```python
from build123d import *

# Parameters (mm, degrees)
F1_DEPTH  = 40
F3_DEPTH  = 30
F4_DEPTH  = 13.8188209357
F6_DEPTH  = 20
F7_R      = 14
F8_DEPTH  = 20
F9_R      = 14
F10_DEPTH = 20


with BuildPart() as f1:
    # F0 (on Top) → F1 (new body)
    with BuildSketch(Plane.XY):
        Polygon((17.6335575688, -24.2705098312), (0, 0), (-30, 0), (-30, -15), (-7.6428817424, -15), (5.4983026531, -33.0872886156), align=None)
        Polygon((9.2705098312, 28.5316954889), (0, 0), (17.6335575688, -24.2705098312), (29.7688124844, -15.4537310469), (16.6276280888, 2.6335575688), (23.5363575757, 23.8964405732), align=None)
        Polygon((-30, 0), (0, 0), (9.2705098312, 28.5316954889), (-4.9953379132, 33.1669504045), (-10.8981379201, 15), (-30, 15), align=None)
    extrude(amount=F1_DEPTH)

    # F2 (on face) → F3 (cut, through all)
    with BuildSketch(Plane(origin=(12.1352549156, 8.8167787844, 0), x_dir=(-0.5877852523, 0.8090169944, 0), z_dir=(0.8090169944, 0.5877852523, 0))):
        Polygon((-30, 26.1811790643), (-7.6428817424, 40), (-30, 40), align=None)
        Polygon((-18.2909047095, 7.2373321675), (-30, 26.1811790643), (-30, 0), (-7.6428817424, 0), (-7.6428817424, 13.8188209357), align=None)
    extrude(amount=-F3_DEPTH, mode=Mode.SUBTRACT)

    # F4 (cut, through all): a face of the model
    f4_faces = [f1.faces().sort_by_distance(p)[0] for p in [
        (-5.1613250879, 7.1039545366, 0),
    ]]
    extrude(f4_faces, amount=-F4_DEPTH, mode=Mode.SUBTRACT)

    # F5 (on face) → F6 (cut)
    with BuildSketch(Plane(origin=(5.8766333563, -8.0884919048, -6.1796670384), x_dir=(0.8660332683, 0.3973019791, 0.303541621), z_dir=(0.4999863781, -0.6881722113, -0.5257686082))):
        with BuildLine():
            ThreePointArc((13.555551142, 11.7065510585), (20.8125243081, 16.7507031763), (23.6020646696, 25.1367388722))
            ThreePointArc((23.6020646696, 25.1367388722), (23.0669801184, 28.9702818755), (21.5026286756, 32.5107863592))
            Line((21.5026286756, 32.5107863592), (5.6485781973, 38.566926686))
            ThreePointArc((5.6485781973, 38.566926686), (-3.4762295905, 30.1325590497), (-2.2984993363, 17.7626913852))
            Line((-2.2984993363, 17.7626913852), (13.555551142, 11.7065510585))
        make_face()
        with BuildLine():
            ThreePointArc((-2.2984993363, 17.7626913852), (4.6062444921, 12.0584446121), (13.555551142, 11.7065510585))
            Line((13.555551142, 11.7065510585), (-2.2984993363, 17.7626913852))
        make_face()
    extrude(amount=-F6_DEPTH, mode=Mode.SUBTRACT)

    # F7 (on face) → F8 (cut)
    with BuildSketch(Plane(origin=(9.2705098312, 28.5316954889, 0), x_dir=(-0.9510565163, 0.3090169944, 0), z_dir=(0.3090169944, 0.9510565163, 0))):
        with Locations((0, 26.9094104679)):
            Circle(F7_R)
    extrude(amount=-F8_DEPTH, mode=Mode.SUBTRACT)

    # F9 (on face) → F10 (cut)
    with BuildSketch(Plane(origin=(-30, 0, 0), x_dir=(0, -1, 0), z_dir=(-1, 0, 0))):
        with Locations((0, 26.9094104679)):
            Circle(F9_R)
    extrude(amount=-F10_DEPTH, mode=Mode.SUBTRACT)


solid = f1.part
```
The listing builds one solid part. Answer for the finished solid, in the listing's coordinates (mm). A direction names the side the tool comes from. Coordinates: 2 decimals unless noted, no trailing zeros. Loops run counter-clockwise (first coordinate to the right, second up) from the corner with the lowest first, then second, coordinate; pieces in that order, holes last. Notation, with made-up numbers: (0.5, -4) -> (46.5, -4) arc R23 ccw to (46.5, 31) -> close; hole circle Ø5 at (89, -5). An arc over 180 degrees is marked (long way). Use one line per item in the form item = value. Start each with the question number.
Item 1: Flat-ended cylindrical pins translate along their axes: pin 1 Ø14.5 at (x, y) = (-1, 11) entering from -Z; pin 2 Ø2 at (x, z) = (17.5, 34.5) entering from -Y; pin 3 Ø5 at (y, z) = (-0.5, 17.5) entering from +X; pin 4 Ø2 at (x, z) = (-8.5, 11) entering from +Y. Find the tip coordinate at first contact, or state that the pin passes through.
Item 2: A tool of negligible diameter and unlimited length cuts with its end or side. For faces 4 (the face through (-19, -15, 27)), 5 (the face through (-7.09, 23.48, 26.67)), 6 (the face through (-10, 0, 27)), from which of +Z, -Z, +X, -X, +Y, -Y can it reach the whole face along a straight path? Write none if from no direction.
Item 3: The part is cut by section A-A on x = -20. Determine the outline of the cut face in (y, z), then the cut area to 3 significant figures.
Item 4: Consider L1, parallel to Z at x = -23, y = 5.5; L2, parallel to Z at x = 13, y = 16.5; L3, parallel to Y at x = 6.5, z = 30.5. Determine where each line is inside the solid, lowest interval first. Write a range as [from, to].
Item 5: The mould has two halves that part along Y. Classify faces 1 (the face through (-20, 14, 27)), 2 (the face through (-4.443, 32.987, 26.848)), 3 (the face through (-2.624, -21.907, 23.389)): released by +Y, released by -Y, zero draft, split by the parting line, or undercut.
Item 6: The part is cut by section B-B on x = 3. Count the separate pieces of the cut face and the enclosed holes in it, then the cut area to 3 significant figures.
Answer key:
q1.pin_1 = 13.82
q1.pin_2 = -9.7
q1.pin_3 = 20.72
q1.pin_4 = through
q2.face_4 = +Z, -Z, -X, -Y
q2.face_5 = none
q2.face_6 = -X
q3.outline = (-15, 13.82) -> (-4.96, 13.82) arc R14 cw to (-4.96, 40) -> (-15, 40) -> close; (4.96, 13.82) -> (15, 13.82) -> (15, 40) -> (4.96, 40) arc R14 cw to start
q3.area = 182 mm2
q4.L1 = [13.82, 14.04], [39.78, 40]
q4.L2 = [13.82, 14.94], [38.88, 40]
q4.L3 = [-23.72, -23.55], [-6.6, 8.4]
q5.face_1 = undercut
q5.face_2 = released by +Y
q5.face_3 = released by -Y
q6.separate_pieces = 5
q6.enclosed_holes = 0
q6.area = 467 mm2
